Model file for the job. Use its own axes, mm. A direction names the side the tool comes from. Give positions to 0.01 mm unless a question says otherwise; leave off trailing zeros. Write each loop counter-clockwise with the first axis right and the second up, starting at its lowest first coordinate (ties: lowest second). Pieces come first, ordered by that corner, then holes. Notation, with made-up numbers: (-12, -37.5) - (43, -37.5) arc R27 cw to (43, -17.5) - close; hole circle Ø6 at (36, 35.5). An arc over 180 degrees is marked (long way). One line per item, written item: value. Start each with the question number.
(1) Cut at A-A, the plane y = 95.5. List the corners of the cut face in (x, z), and give its area (3 significant figures).
(2) 3-axis set-ups, long thin cutter, end or side, ignore diameter. For faces 5 (the face through (20.185, 173, 9)), 6 (the face through (7.835, 18, 9)), 7 (the face through (28.35, 146, 5)), 8 (the face through (14, 148, 10.3)), 9 (the face through (42, 181.225, 9)): which of +Z, -Z, +X, -X, +Y, -Y reach the whole face in a straight line?
(3) Drop flat-ended pins along their axis: P1, Ø1.2, axis at y = 145, z = 9.5, coming from the -X side; P2, Ø3, axis at x = 14, z = 3.5, coming from the +Y side (3 decimals); P3, Ø4.5, axis at x = 52, y = 4, coming from the -Z side; P4, Ø1.5, axis at x = 40.5, y = 107.5, coming from the +Z side. Give the stop position or say it passes through.
(4) Cut at B-B, the plane x = 4. List the corners of the cut face in (y, z).
(5) Probe L1, parallel to Y at x = 13, z = 7.75 (3 decimals); L2, parallel to Y at x = 12, z = 15.75 (3 decimals); L3, parallel to Y at x = 36, z = 1.5 (3 decimals). List the from-to ranges inside material, lowest first.
(6) Mould opens along X. For faces 1 (the face through (55.65, 146, 5)), 2 (the face through (6.385, 4.751, 0.641)), 3 (the face through (42, 164.225, 9)), 4 (the face through (13, 90, 11)) say: pulls with the +X half, pulls with the -X half, needs draft (parallel to the pull), parting line crosses it, or undercut.
(7) Cut at D-D, the plane y = 184. List the corners of the cut face in (x, z).
(8) Cut at C-C, the plane y = 4. List the corners of the cut face in (x, z), and give its area (3 significant figures).
from build123d import *

# Parameters (mm, degrees)
SKETCH1_R                = 2.5
SKETCH1_W                = 12.35
SKETCH1_H                = 17
BOSS_EXTRUDE1_DEPTH      = 1.3
BOSS_EXTRUDE2_DEPTH      = 15
BOSS_EXTRUDE2_DEPTH_BACK = 1.3
SKETCH2_W                = 12.35
SKETCH2_H                = 17
SKETCH3_W                = 27.3
SKETCH3_H                = 27.8
BOSS_EXTRUDE3_DEPTH      = 7.5
SKETCH4_W                = 25
SKETCH4_H                = 13
BOSS_EXTRUDE4_DEPTH      = 1.5
SKETCH5_W                = 9
SKETCH5_H                = 75
SKETCH5_W_2              = 2.5
SKETCH5_H_2              = 65
BOSS_EXTRUDE5_DEPTH      = 6.5
SKETCH7_W                = 1
SKETCH7_H                = 1
SKETCH7_H_2              = 65
BOSS_EXTRUDE6_DEPTH      = 6.5


with BuildPart() as part:
    # Sketch1 → Boss-Extrude1 (new body)
    with BuildSketch(Plane.XY):
        Polygon((0, 200), (0, 0), (3.731641176, 0), (10.2, 0), (28, 0), (38.2, 0), (56, 0), (56, 200), align=None)
        with Locations((4, 4)):
            Circle(SKETCH1_R, mode=Mode.SUBTRACT)
        Polygon((20.185, 9.125), (10.2, 9.125), (7.835, 9.125), (7.835, 26.125), (20.185, 26.125), align=None, mode=Mode.SUBTRACT)
        with Locations((14.01, 35.625)):
            Rectangle(SKETCH1_W, SKETCH1_H, mode=Mode.SUBTRACT)
        Polygon((48.185, 9.125), (38.2, 9.125), (35.835, 9.125), (35.835, 26.125), (48.185, 26.125), align=None, mode=Mode.SUBTRACT)
        with Locations((52, 4)):
            Circle(SKETCH1_R, mode=Mode.SUBTRACT)
        with Locations((42.01, 35.625)):
            Rectangle(SKETCH1_W, SKETCH1_H, mode=Mode.SUBTRACT)
        Polygon((20.185, 164.225), (10.2, 164.225), (7.835, 164.225), (7.835, 181.225), (20.185, 181.225), align=None, mode=Mode.SUBTRACT)
        with BuildLine():
            ThreePointArc((30.5, 175), (29.767766953, 173.232233047), (28, 172.5))
            ThreePointArc((28, 172.5), (26.232233047, 176.767766953), (30.5, 175))
        make_face(mode=Mode.SUBTRACT)
        Polygon((48.185, 164.225), (38.2, 164.225), (35.835, 164.225), (35.835, 181.225), (48.185, 181.225), align=None, mode=Mode.SUBTRACT)
    extrude(amount=BOSS_EXTRUDE1_DEPTH)

    # Sketch2 → Boss-Extrude2 (add, two sides: drawn at the far end of the back side and taken through both)
    with BuildSketch(Plane.XY.offset(1.3).offset(-BOSS_EXTRUDE2_DEPTH_BACK)):
        with Locations((14.01, 172.725)):
            Rectangle(SKETCH2_W, SKETCH2_H)
        with Locations((42.01, 172.725)):
            Rectangle(SKETCH2_W, SKETCH2_H)
        with Locations((42.01, 35.625)):
            Rectangle(SKETCH2_W, SKETCH2_H)
        with Locations((42.01, 17.625)):
            Rectangle(SKETCH2_W, SKETCH2_H)
        with Locations((14.01, 17.625)):
            Rectangle(SKETCH2_W, SKETCH2_H)
        with Locations((14.01, 35.625)):
            Rectangle(SKETCH2_W, SKETCH2_H)
    extrude(amount=BOSS_EXTRUDE2_DEPTH + BOSS_EXTRUDE2_DEPTH_BACK)

    # Sketch3 → Boss-Extrude3 (add)
    with BuildSketch(Plane.XY.offset(1.3)):
        with Locations((14, 146.1)):
            Rectangle(SKETCH3_W, SKETCH3_H)
        with Locations((42, 146.1)):
            Rectangle(SKETCH3_W, SKETCH3_H)
    extrude(amount=BOSS_EXTRUDE3_DEPTH)

    # Sketch4 → Boss-Extrude4 (add)
    with BuildSketch(Plane.XY.offset(8.8)):
        with Locations((14, 147.7)):
            Rectangle(SKETCH4_W, SKETCH4_H)
        with Locations((42, 147.7)):
            Rectangle(SKETCH4_W, SKETCH4_H)
    extrude(amount=BOSS_EXTRUDE4_DEPTH)

    # Sketch5 → Boss-Extrude5 (add)
    # profile 1 of 2: a face of its own
    with BuildSketch(Plane.XY.offset(1.3)):
        with Locations((14, 90)):
            Rectangle(SKETCH5_W, SKETCH5_H)
        with Locations((14, 89.5)):
            Rectangle(SKETCH5_W_2, SKETCH5_H_2, mode=Mode.SUBTRACT)
    # profile 2 of 2: a face of its own
    with BuildSketch(Plane.XY.offset(1.3)):
        with Locations((42, 90)):
            Rectangle(SKETCH5_W, SKETCH5_H)
        with Locations((42, 89.5)):
            Rectangle(SKETCH5_W_2, SKETCH5_H_2, mode=Mode.SUBTRACT)
    extrude(amount=BOSS_EXTRUDE5_DEPTH)

    # Sketch7 → Boss-Extrude6 (add)
    with BuildSketch(Plane.XY.offset(7.8)):
        with Locations((13.5, 122.5)):
            Rectangle(SKETCH7_W, SKETCH7_H)
        with Locations((14.5, 122.5)):
            Rectangle(SKETCH7_W, SKETCH7_H)
        with Locations((13.5, 89.5)):
            Rectangle(SKETCH7_W, SKETCH7_H_2)
        with Locations((14.5, 89.5)):
            Rectangle(SKETCH7_W, SKETCH7_H_2)
        with Locations((14.5, 56.5)):
            Rectangle(SKETCH7_W, SKETCH7_H)
        with Locations((13.5, 56.5)):
            Rectangle(SKETCH7_W, SKETCH7_H)
    extrude(amount=BOSS_EXTRUDE6_DEPTH)


solid = part.part
Answers follow:
1. outline: (0, 0) - (56, 0) - (56, 1.3) - (46.5, 1.3) - (46.5, 7.8) - (43.25, 7.8) - (43.25, 1.3) - (40.75, 1.3) - (40.75, 7.8) - (37.5, 7.8) - (37.5, 1.3) - (18.5, 1.3) - (18.5, 7.8) - (15.25, 7.8) - (15.25, 1.3) - (12.75, 1.3) - (12.75, 7.8) - (9.5, 7.8) - (9.5, 1.3) - (0, 1.3) - close; (13, 7.8) - (15, 7.8) - (15, 14.3) - (13, 14.3) - close
1. area: 170 mm²
2. face 5: +Z, +Y
2. face 6: +Z, -X, -Y
2. face 7: +Z, +Y, -Y
2. face 8: +Z, +X, -X
2. face 9: +Z, +X, -X, +Y
3. P1: stops at x = 1.5
3. P2: stops at y = 181.225
3. P3: passes through
3. P4: stops at z = 7.8
4. outline: (0, 0) - (1.5, 0) - (1.5, 1.3) - (0, 1.3) - close; (6.5, 0) - (200, 0) - (200, 1.3) - (160, 1.3) - (160, 8.8) - (154.2, 8.8) - (154.2, 10.3) - (141.2, 10.3) - (141.2, 8.8) - (132.2, 8.8) - (132.2, 1.3) - (6.5, 1.3) - close
5. L1: y = 9.125 to 26.125, 27.125 to 44.125, 52.5 to 57, 122 to 127.5, 132.2 to 160, 164.225 to 181.225
5. L2: y = 9.125 to 26.125, 27.125 to 44.125, 164.225 to 181.225
5. L3: y = 9.125 to 26.125, 27.125 to 44.125, 132.2 to 160, 164.225 to 181.225
6. face 1: pulls with the +X half
6. face 2: undercut
6. face 3: needs draft
6. face 4: pulls with the -X half
7. outline: (0, 0) - (56, 0) - (56, 1.3) - (0, 1.3) - close
8. outline: (0, 0) - (1.5, 0) - (1.5, 1.3) - (0, 1.3) - close; (6.5, 0) - (49.5, 0) - (49.5, 1.3) - (6.5, 1.3) - close; (54.5, 0) - (56, 0) - (56, 1.3) - (54.5, 1.3) - close
8. area: 59.8 mm²
